Design review of the part shown in the three views and the two pictorial views. Dimensions are in mm from the part's minimum x, y and z. A direction names the side the tool comes from. Round coordinates to 2 decimals unless told otherwise and drop trailing zeros. Order: outer loops, then holes, each group sorted by start corner. A loop starts at its lowest first (then second) coordinate and runs counter-clockwise, first axis right, second up.
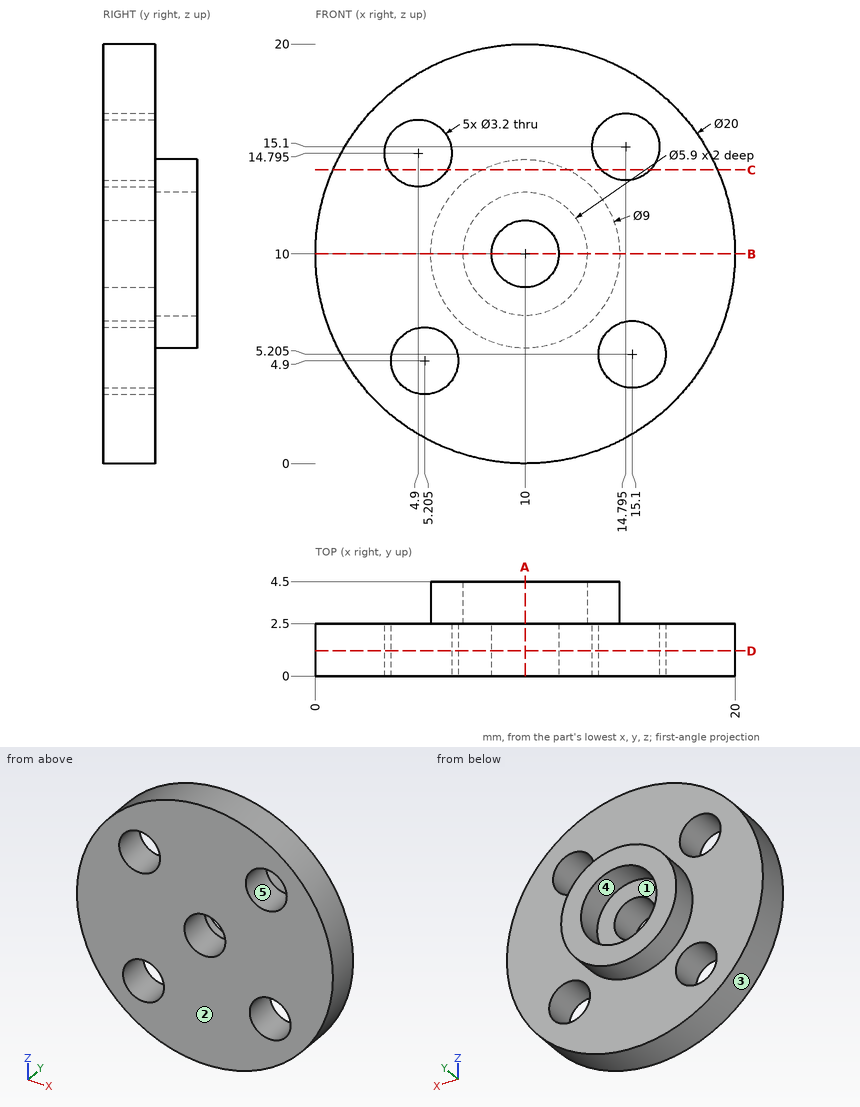
1) Clearance check with flat-ended pins moving along their axes: P1, Ø5.5, axis at x = 10, z = 10, coming from the +Y side; P2, Ø2, axis at x = 18, y = 2, coming from the +Z side; P3, Ø2, axis at x = 16, y = 2, coming from the +Z side; P4, Ø3.5, axis at x = 15.1, z = 5.2, coming from the -Y side. State where each tip first meets the part, or that it passes through.
Results:
P1: stops at y = 2.5
P2: stops at z = 17.14
P3: stops at z = 18.66
P4: stops at y = 0
2) The part is to be moulded in two halves that separate along Z. For the marked faces 1, 2 and 3, say which applies: released by +Z, released by -Z, zero draft, split by the parting line, or undercut.
Results:
face 1: undercut
face 2: zero draft
face 3: split by the parting line
3) Take a section at A-A on x = 10. Give the boundary of the cut face in (y, z), plus the area to 3 significant figures.
Results:
outline: (0, 0) - (2.5, 0) - (2.5, 5.5) - (4.5, 5.5) - (4.5, 7.05) - (2.5, 7.05) - (2.5, 8.4) - (0, 8.4) - close; (0, 11.6) - (2.5, 11.6) - (2.5, 12.95) - (4.5, 12.95) - (4.5, 14.5) - (2.5, 14.5) - (2.5, 20) - (0, 20) - close
area: 48.2 mm2
4) To check wall thickness, follow line 1 along X through (y, z) = (0.7, 6.25) (1 decimal); line 2 along Z through (x, y) = (10, 2.95); line 3 along Z through (x, y) = (14, 0.55) (1 decimal). State the ranges of each line that lie inside material, in increasing order.
Results:
line 1: x = 0.7 to 4.3, 6.1 to 13.9, 16.3 to 19.3
line 2: z = 5.5 to 7.05, 12.95 to 14.5
line 3: z = 0.8 to 4, 6.4 to 13.7, 16.5 to 19.2
5) For the marked faces 4 and 5, list the 3-axis set-ups (+Z, -Z, +X, -X, +Y, -Y) from which the entire face can be reached by the end or side of a thin tool; tool diameter is ignored.
Results:
face 4: +Y
face 5: +Y, -Y
6) Take a section at B-B on z = 10. Give the boundary of the cut face in (x, y), plus the area to 3 significant figures.
Results:
outline: (0, 0) - (8.4, 0) - (8.4, 2.5) - (7.05, 2.5) - (7.05, 4.5) - (5.5, 4.5) - (5.5, 2.5) - (0, 2.5) - close; (11.6, 0) - (20, 0) - (20, 2.5) - (14.5, 2.5) - (14.5, 4.5) - (12.95, 4.5) - (12.95, 2.5) - (11.6, 2.5) - close
area: 48.2 mm2
7) Take a section at C-C on z = 14. Give the boundary of the cut face in (x, y) (1 decimal).
Results:
outline: (0.8, 0) - (3.5, 0) - (3.5, 2.5) - (0.8, 2.5) - close; (6.3, 0) - (13.6, 0) - (13.6, 2.5) - (12.1, 2.5) - (12.1, 4.5) - (7.9, 4.5) - (7.9, 2.5) - (6.3, 2.5) - close; (16, 0) - (19.2, 0) - (19.2, 2.5) - (16, 2.5) - close
8) Take a section at D-D on y = 1.2. Give the boundary of the cut face in (x, z) (1 decimal).
Results:
outline: circle Ø20 at (10, 10); hole circle Ø3.2 at (4.9, 14.8); hole circle Ø3.2 at (5.2, 4.9); hole circle Ø3.2 at (10, 10); hole circle Ø3.2 at (14.8, 15.1); hole circle Ø3.2 at (15.1, 5.2)
